Model file for the job. Use its own axes, mm. A direction names the side the tool comes from. Round coordinates to 2 decimals unless told otherwise and drop trailing zeros. Write each loop counter-clockwise with the first axis right and the second up, starting at its lowest first coordinate (ties: lowest second). Pieces come first, ordered by that corner, then holes. Notation, with made-up numbers: (61.25, -35.75) - (110.25, -35.75) arc R10 ccw to (110.25, -27.75) - close; hole circle Ø8 at (54, -39.5). An arc over 180 degrees is marked (long way). One line per item, written item: value.
from build123d import *

# Parameters (mm, degrees)
SKETCH_1_W          = 20.5
SKETCH_1_H          = 35
EXTRUDE_1_DEPTH     = 17.8
SKETCH_3_R          = 3
EXTRUDE_2_DEPTH     = 2
SKETCH_4_R          = 5
EXTRUDE_3_DEPTH     = 3
SKETCH_5_W          = 20.5
SKETCH_5_H          = 25
CUT_EXTRUDE_1_DEPTH = 6.5
FILLET_1_R          = 1
SKETCH_6_W          = 12
SKETCH_6_H          = 18
EXTRUDE_4_DEPTH     = 4


with BuildPart() as part:
    # 草圖1 → 填料-伸長1 (new body)
    with BuildSketch(Plane.XY):
        Rectangle(SKETCH_1_W, SKETCH_1_H)
    extrude(amount=EXTRUDE_1_DEPTH)

    # 草圖3 → 填料-伸長2 (add)
    with BuildSketch(Plane.XZ.offset(17.5)):
        with Locations((0, 8.9)):
            Circle(SKETCH_3_R)
    extrude(amount=EXTRUDE_2_DEPTH)

    # 草圖4 → 填料-伸長3 (add)
    with BuildSketch(Plane.XZ.offset(19.5)):
        with Locations((0, 8.9)):
            Circle(SKETCH_4_R)
    extrude(amount=EXTRUDE_3_DEPTH)

    # 草圖5 → 除料-伸長1 (cut)
    with BuildSketch(Plane.XY.offset(17.8)):
        with Locations((0, 5)):
            Rectangle(SKETCH_5_W, SKETCH_5_H)
    extrude(amount=-CUT_EXTRUDE_1_DEPTH, mode=Mode.SUBTRACT)

    # 圓角1
    fillet_1_edges = [part.edges().sort_by_distance(p)[0] for p in [
        (0, -17.5, 17.8),
        (-5, -22.5, 8.9),
        (-10.25, -12.5, 17.8),
        (-10.25, 17.5, 5.65),
        (10.25, 17.5, 5.65),
        (-10.25, 5, 11.3),
        (-10.25, -7.5, 14.55),
        (0, 17.5, 11.3),
        (10.25, 5, 11.3),
        (0, -7.5, 11.3),
        (10.25, -7.5, 14.55),
        (0, -7.5, 17.8),
        (10.25, -12.5, 17.8),
        (10.25, -17.5, 8.9),
        (-10.25, -17.5, 8.9),
    ]]
    fillet(fillet_1_edges, radius=FILLET_1_R)

    # 草圖6 → 填料-伸長4 (add)
    with BuildSketch(Plane.XY.offset(11.3)):
        with Locations((0, 5)):
            Rectangle(SKETCH_6_W, SKETCH_6_H)
    extrude(amount=EXTRUDE_4_DEPTH)


solid = part.part
1. Mould opens along Y. For faces 1 (the face through (9.949, -17.215, 8.518)), 2 (the face through (9.949, -12.444, 17.515)), 3 (the face through (-2, -17.5, 6)) say: released by +Y, released by -Y, zero draft, split by the parting line, or undercut.
Report:
face 1: released by -Y
face 2: zero draft
face 3: undercut
2. Band-saw the part on A-A on x = 0. Write the cut outline in (y, z), plus the area to 3 significant figures.
Report:
outline: (-22.5, 4.9) arc R1 ccw to (-21.5, 3.9) - (-19.5, 3.9) - (-19.5, 5.9) - (-17.5, 5.9) - (-17.5, 0) - (17.5, 0) - (17.5, 10.3) arc R1 ccw to (16.5, 11.3) - (14, 11.3) - (14, 15.3) - (-4, 15.3) - (-4, 11.3) - (-6.5, 11.3) arc R1 cw to (-7.5, 12.3) - (-7.5, 16.8) arc R1 ccw to (-8.5, 17.8) - (-16.5, 17.8) arc R1 ccw to (-17.5, 16.8) - (-17.5, 11.9) - (-19.5, 11.9) - (-19.5, 13.9) - (-21.5, 13.9) arc R1 ccw to (-22.5, 12.9) - close
area: 574 mm²
3. Band-saw the part on D-D on x = 7. Write the cut outline in (y, z).
Report:
outline: (-17.5, 0) - (17.5, 0) - (17.5, 10.3) arc R1 ccw to (16.5, 11.3) - (-6.5, 11.3) arc R1 cw to (-7.5, 12.3) - (-7.5, 16.8) arc R1 ccw to (-8.5, 17.8) - (-16.5, 17.8) arc R1 ccw to (-17.5, 16.8) - close
4. Wall check: probe 1 along Y at (x, z) = (4, 14.5); probe 2 along Y at (x, z) = (3.75, 16.5); probe 3 along Z at (x, y) = (-8.75, 2). Give the ranges that are in metal, low to high. Write a range as [from, to].
Report:
probe 1: [-17.5, -7.5], [-4, 14]
probe 2: [-17.5, -7.5]
probe 3: [0, 11.3]
5. Drop flat-ended pins along their axis: pin 1 (12 mm diameter, centred on x = 4.5, y = -9, fed in from -Z); pin 2 (3 mm diameter, centred on y = 2, z = 13, fed in from +X); pin 3 (5 mm diameter, centred on x = -1.5, y = 10, fed in from +Z); pin 4 (1.3 mm diameter, centred on x = 1, z = 14, fed in from +Y). Give the stop position or say it passes through.
Report:
pin 1: z = 0
pin 2: x = 6
pin 3: z = 15.3
pin 4: y = 14
6. Band-saw the part on B-B on y = 4. Write the cut outline in (x, z), plus the area to 3 significant figures.
Report:
outline: (-10.25, 0) - (10.25, 0) - (10.25, 10.3) arc R1 ccw to (9.25, 11.3) - (6, 11.3) - (6, 15.3) - (-6, 15.3) - (-6, 11.3) - (-9.25, 11.3) arc R1 ccw to (-10.25, 10.3) - close
area: 279 mm²
7. Tool access for faces 4 (the face through (-6, 5, 13)), 5 (the face through (0, -4, 13)), 6 (the face through (6, 5, 13)): list every direction of +Z, -Z, +X, -X, +Y, -Y with a clear straight run to the whole face (end or side of a thin tool).
Report:
face 4: +Z, -X, +Y
face 5: +Z, +X, -X
face 6: +Z, +X, +Y
8. Band-saw the part on C-C on z = 8.9. Write the cut outline in (x, y), plus the area to 3 significant figures.
Report:
outline: (-10.25, -16.5) arc R1 ccw to (-9.25, -17.5) - (-3, -17.5) - (-3, -19.5) - (-5, -19.5) - (-5, -21.5) arc R1 ccw to (-4, -22.5) - (4, -22.5) arc R1 ccw to (5, -21.5) - (5, -19.5) - (3, -19.5) - (3, -17.5) - (9.25, -17.5) arc R1 ccw to (10.25, -16.5) - (10.25, 16.5) arc R1 ccw to (9.25, 17.5) - (-9.25, 17.5) arc R1 ccw to (-10.25, 16.5) - close
area: 758 mm²
